Source: CAD feature listing. Evaluate the final solid. Frame: model axes, mm. Face numbers are marked on the shaded views. Coordinates: 2 decimals unless noted, no trailing zeros. Order: outer loops, then holes, each group sorted by start corner. A loop starts at its lowest first (then second) coordinate and runs counter-clockwise, first axis right, second up.
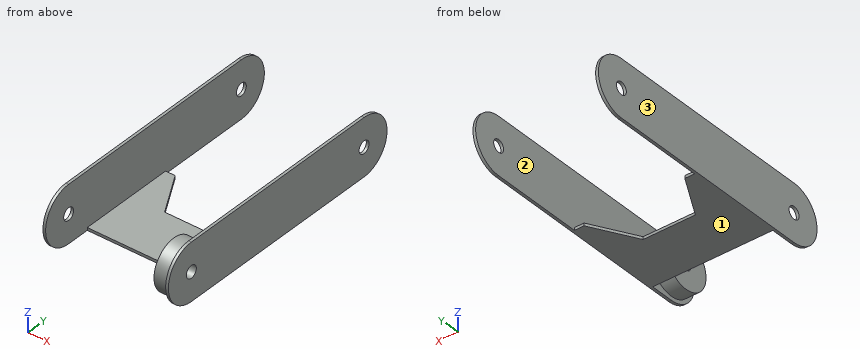
Autodesk Inventor part; units mm, degrees
ref_plane "Work Plane2" through (64.7065, 0, 0) normal (1, 0, 0) x (0, 0, -1)
ref_plane "YZ Plane" through (0, 0, 0) normal (1, 0, 0) x (0, 1, 0)
ref_plane "XZ Plane" through (0, 0, 0) normal (0, 1, 0) x (-1, 0, 0)
sketch "Sketch1" plane through (0, 0, 0) normal (1, 0, 0) x (0, 1, 0)
  circle A0 centre (0, 0) radius 29.3688
  circle A1 centre (220.6625, 0) radius 29.3688
  line L0 (220.6625, -29.3688) -> (0, -29.3688)
  line L1 (220.6625, 29.3687) -> (0, 29.3687)
  line L2 (0, 0) -> (220.6625, 0) construction
  dimension "d0" = 58.7375
  dimension "d1" = 220.6625
extrude "Extrusion1" add sketch "Sketch1" along normal blind 2.794
ref_plane "Work Plane2" through (64.7065, 0, 0) normal (1, 0, 0) x (0, 0, -1)
ref_plane "Work Plane1" through (126.619, 0, 0) normal (1, 0, 0) x (0, 0, -1)
mirror "Mirror1" about plane through (64.7065, 0, 0) normal (1, 0, 0) of "Extrusion1"
sketch "Sketch2" plane through (2.794, 0, 0) normal (1, 0, 0) x (0, 0, -1)
  line L0 (29.3688, 0) -> (29.3688, 220.6625)
  line L1 (29.3688, 123.825) -> (26.5748, 123.825)
  line L2 (26.5748, 123.825) -> (26.5748, 23.8125)
  line L3 (26.5748, 23.8125) -> (29.3688, 23.8125)
  line L4 (29.3688, 23.8125) -> (29.3688, 123.825)
  arc A0 (29.3688, 220.6625) -> (-29.3687, 220.6625) centre (0, 220.6625) ccw
  point P0 (0, 0)
  dimension "d6" = 100.0125
  dimension "d7" = 2.794
  dimension "d8" = 96.8375
extrude "Extrusion2" add sketch "Sketch2" along normal up to next
sketch "Sketch3" plane through (0, 0, -29.3688) normal (0, 0, -1) x (-1, 0, 0)
  line L0 (0, 0) -> (0, 220.6625)
  line L1 (0, 220.6625) -> (-2.794, 220.6625)
  line L2 (-2.794, 123.825) -> (-2.794, 220.6625)
  line L3 (-2.794, 123.825) -> (-126.619, 123.825)
  line L4 (-126.619, 123.825) -> (-126.619, 220.6625)
  line L5 (-129.413, 220.6625) -> (-126.619, 220.6625)
  line L6 (-129.413, 0) -> (-129.413, 220.6625)
  line L7 (-129.413, 0) -> (-126.619, 0)
  line L8 (-126.619, 0) -> (-126.619, 23.8125)
  line L9 (-2.794, 23.8125) -> (-126.619, 23.8125)
  line L10 (-2.794, 0) -> (-2.794, 23.8125)
  line L11 (0, 0) -> (-2.794, 0)
  line L12 (-116.713, 123.825) -> (-91.694, 79.375)
  line L13 (-91.694, 79.375) -> (-37.719, 79.375)
  line L14 (-37.719, 79.375) -> (-12.7, 123.825)
  line L15 (-64.7065, 79.375) -> (-64.7065, 123.825)
  point P0 (0, 0)
  dimension "d11" = 12.7
  dimension "d12" = 12.7
  dimension "d13" = 53.975
  dimension "d14" = 44.45
extrude "Extrusion3" cut sketch "Sketch3" against normal blind 2.794 contours L14 L13 L15 L3 | L15 L13 L12 L3
sketch "Sketch5" plane through (126.619, 0, 29.3687) normal (-1, 0, 0) x (0, 0, 1)
  circle A0 centre (-29.3687, 0) radius 25.4
  dimension "d21" = 50.8
extrude "Extrusion5" add sketch "Sketch5" along normal blind 15.24
sketch "Sketch4" plane through (129.413, 0, 29.3687) normal (1, 0, 0) x (0, 0, -1)
  arc A0 (58.7375, 220.6625) -> (0, 220.6625) centre (29.3687, 220.6625) ccw
  circle A1 centre (29.3687, 220.6625) radius 6.35
  circle A2 centre (29.3687, 0) radius 6.35
  dimension "d17" = 12.7
  dimension "d18" = 12.7
extrude "Extrusion4" cut sketch "Sketch4" against normal through all
properties part number "Top_Arm" material "Aluminum 6061"
Q1. Section query C-C on z = 14. Output: boundary loops of the cut face in (x, y).
Solutions:
outline: (0, -25.82) - (2.79, -25.82) - (2.79, 246.48) - (0, 246.48) - close; (111.38, -21.19) - (126.62, -21.19) - (126.62, -25.82) - (129.41, -25.82) - (129.41, 246.48) - (126.62, 246.48) - (126.62, 21.19) - (111.38, 21.19) - close
Q2. Section query A-A on z = 0. Output: boundary loops of the cut face in (x, y), plus the area to 3 significant figures.
Solutions:
outline: (0, -29.37) - (2.79, -29.37) - (2.79, -6.35) - (0, -6.35) - close; (0, 6.35) - (2.79, 6.35) - (2.79, 214.31) - (0, 214.31) - close; (0, 227.01) - (2.79, 227.01) - (2.79, 250.03) - (0, 250.03) - close; (111.38, -25.4) - (126.62, -25.4) - (126.62, -29.37) - (129.41, -29.37) - (129.41, -6.35) - (111.38, -6.35) - close; (111.38, 6.35) - (129.41, 6.35) - (129.41, 214.31) - (126.62, 214.31) - (126.62, 25.4) - (111.38, 25.4) - close; (126.62, 227.01) - (129.41, 227.01) - (129.41, 250.03) - (126.62, 250.03) - close
area: 2,000 mm2
Q3. Section query B-B on y = 157.5. Output: boundary loops of the cut face in (x, z).
Solutions:
outline: (0, -29.37) - (2.79, -29.37) - (2.79, 29.37) - (0, 29.37) - close; (126.62, -29.37) - (129.41, -29.37) - (129.41, 29.37) - (126.62, 29.37) - close
Q4. Material intervals for line 1 along Y through (x, z) = (1.4, 0); line 2 along X through (y, z) = (231.5, 3.5); line 3 along X through (y, z) = (-7, 18), sorted ascending.
Solutions:
line 1: y = -29.37 to -6.35, 6.35 to 214.31, 227.01 to 250.03
line 2: x = 0 to 2.79, 126.62 to 129.41
line 3: x = 0 to 2.79, 111.38 to 129.41
Q5. Pin query (flat end, axial travel): P1, Ø2, axis at x = 10, z = -28, coming from the +Y side (3 decimals); P2, Ø1.4, axis at x = 88.5, z = -28, coming from the -Y side; P3, Ø1.4, axis at x = 68, z = -28, coming from the +Y side (3 decimals). Return the tip coordinate at first contact, or that it passes through.
Solutions:
P1: stops at y = 123.825
P2: stops at y = 23.81
P3: stops at y = 79.375
Q6. Pull-direction query (X, two-part tool) for the marked faces 1, 2 and 3; classes: pulls with the +X half, pulls with the -X half, needs draft (parallel to the pull), parting line crosses it, or undercut.
Solutions:
face 1: needs draft
face 2: undercut
face 3: pulls with the -X half
Q7. Section query D-D on y = 72. Output: boundary loops of the cut face in (x, z).
Solutions:
outline: (0, -29.37) - (129.41, -29.37) - (129.41, 29.37) - (126.62, 29.37) - (126.62, -26.57) - (2.79, -26.57) - (2.79, 29.37) - (0, 29.37) - close
